Autodesk Inventor part; units mm, degrees
ref_plane "YZ Plane" through (0, 0, 0) normal (1, 0, 0) x (0, 1, 0)
ref_plane "XZ Plane" through (0, 0, 0) normal (0, 1, 0) x (-1, 0, 0)
ref_plane "XY Plane" through (0, 0, 0) normal (0, 0, 1) x (1, 0, 0)
sketch "Sketch1" plane through (0, 0, 0) normal (0, 0, 1) x (1, 0, 0)
  line L0 (-21.6696, 43.0812) -> (79.9304, 43.0812)
  line L1 (79.9304, 43.0812) -> (79.9304, -20.4188)
  line L2 (79.9304, -20.4188) -> (-21.6696, -20.4188)
  line L3 (-21.6696, -20.4188) -> (-21.6696, 43.0812)
  point P0 (0, 0)
  dimension "d0" = 101.6
  dimension "d1" = 63.5
extrude "Extrusion1" add sketch "Sketch1" along normal blind 7.9375
sketch "Sketch3" plane through (0, 0, 7.9375) normal (0, 0, 1) x (1, 0, 0)
  line L0 (-21.6696, 43.0812) -> (79.9304, 43.0812)
  line L1 (-21.6696, -20.4188) -> (-21.6696, 43.0812)
  point P0 (0, 0)
  point P1 (29.1304, 11.3312)
  dimension "d15" = 31.75
  dimension "d16" = 50.8
hole "Hole2" at (29.1304, 11.3312, 7.9375) direction (0, 0, -1) diameter 50.8 end through all
sketch "Sketch4" plane through (0, 0, 7.9375) normal (0, 0, 1) x (1, 0, 0)
  line L0 (-21.6696, -20.4188) -> (-21.6696, 43.0812)
  line L1 (79.9304, -20.4188) -> (-21.6696, -20.4188)
  point P0 (0, 0)
  point P1 (10.0804, 36.7312)
  point P2 (10.0804, -14.0688)
  point P3 (48.1804, 36.7312)
  point P4 (48.1804, -14.0688)
  dimension "d24" = 50.8
  dimension "d25" = 6.35
  dimension "d26" = 38.1
  dimension "d27" = 31.75
  dimension "d28" = 31.75
hole "Hole3" at (10.0804, 36.7312, 7.9375) at (10.0804, -14.0688, 7.9375) at (48.1804, 36.7312, 7.9375) at (48.1804, -14.0688, 7.9375) direction (0, 0, -1) diameter 3.9624 end through all
sketch "Sketch5" plane through (0, 0, 7.9375) normal (0, 0, 1) x (1, 0, 0)
  line L0 (79.9304, 43.0812) -> (79.9304, -20.4188)
  line L1 (-21.6696, 43.0812) -> (79.9304, 43.0812)
  line L2 (-21.6696, -20.4188) -> (-21.6696, 43.0812)
  line L3 (79.9304, -20.4188) -> (-21.6696, -20.4188)
  point P0 (0, 0)
  point P1 (-18.1136, 39.5252)
  point P2 (-18.1136, -16.8628)
  point P3 (76.3744, -16.8628)
  point P4 (76.3744, 39.5252)
  point P5 (-18.1136, 11.3312)
  point P6 (76.3744, 11.3312)
  dimension "d36" = 3.556
  dimension "d37" = 3.556
  dimension "d38" = 3.556
  dimension "d39" = 3.556
  dimension "d47" = 3.556
  dimension "d48" = 3.556
  dimension "d49" = 3.556
  dimension "d50" = 3.556
  dimension "d51" = 3.556
  dimension "d52" = 3.556
  dimension "d66" = 94.488
  dimension "d67" = 56.388
hole "Hole4" at (-18.1136, 39.5252, 7.9375) at (-18.1136, -16.8628, 7.9375) at (76.3744, -16.8628, 7.9375) at (76.3744, 39.5252, 7.9375) at (-18.1136, 11.3312, 7.9375) at (76.3744, 11.3312, 7.9375) direction (0, 0, -1) diameter 4.318 end through all counterbore diameter 6.985 counterbore depth 4.1656
sketch "Sketch6" plane through (0, 0, 7.9375) normal (0, 0, 1) x (1, 0, 0)
  line L0 (79.9304, 43.0812) -> (79.9304, -20.4188)
  line L1 (-21.6696, 43.0812) -> (79.9304, 43.0812)
  line L2 (-21.6696, -20.4188) -> (-21.6696, 43.0812)
  line L3 (79.9304, -20.4188) -> (-21.6696, -20.4188)
  point P0 (0, 0)
  point P1 (-8.9696, 30.3812)
  point P2 (-8.9696, -7.7188)
  point P3 (67.2304, 30.3812)
  point P4 (67.2304, -7.7188)
  dimension "d53" = 12.7
  dimension "d54" = 12.7
  dimension "d55" = 12.7
  dimension "d56" = 12.7
  dimension "d64" = 12.7
  dimension "d65" = 12.7
hole "Hole5" at (-8.9696, 30.3812, 7.9375) at (-8.9696, -7.7188, 7.9375) at (67.2304, 30.3812, 7.9375) at (67.2304, -7.7188, 7.9375) direction (0, 0, -1) diameter 6.4008 end through all
properties part number "JF-AT-JC0014" material "Aluminum-6061 (Anodized Black)"
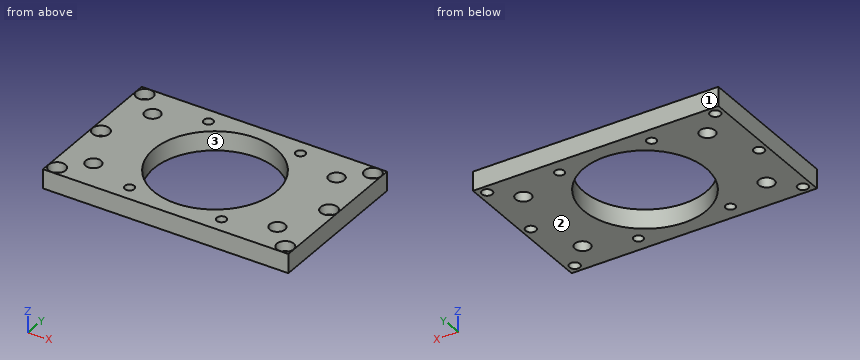
Model file for the job. Use its own axes, mm. Face numbers are marked on the shaded views. Give positions to 0.01 mm unless a question says otherwise; leave off trailing zeros. Order: outer loops, then holes, each group sorted by start corner. A loop starts at its lowest first (then second) coordinate and runs counter-clockwise, first axis right, second up. Notation, with made-up numbers: M 16,-7.75 L 23,-7.75 A12 cw 23,3.25 Z; hole C 9,88 d3. An arc over 180 degrees is marked long. Put each result on its own line as item: value. Start each with the question number.
(1) Pull direction Y, two halves, no side cores. Call the marked faces 1, 2 and 3: released by +Y, released by -Y, zero draft, split by the parting line, or undercut.
(2) Band-saw the part on A-A on y = 11.5. Give the cut face in (x, z).
(3) Band-saw the part on C-C on x = 24. Give the cut face in (y, z).
(4) Band-saw the part on B-B on z = 5.25. Count the separate pieces of the cut face and the enclosed holes in it, then the cut area to 3 significant figures.
(5) Band-saw the part on D-D on y = 20.5. Give the cut face in (x, z).
(6) Pin check, flat tips, straight feed: pin 1 Ø2 at (x, y) = (77.5, -15) entering from +Z; pin 2 Ø3 at (x, y) = (10.08, 36.73) entering from -Z. Stop position of each tip, or through.
(7) Drill centre lines: L1, parallel to X at y = 9, z = 7; L2, parallel to X at y = -15, z = 5.5; L3, parallel to X at y = -5.5, z = 1. Where is each one in solid material? Low to high. Write a range as [from, to].
Results below:
1. face 1: released by +Y
1. face 2: zero draft
1. face 3: undercut
2. outline: M -21.67,0 L -20.27,0 L -20.27,3.77 L -21.6,3.77 L -21.6,7.94 L -21.67,7.94 Z; M -15.96,0 L 3.73,0 L 3.73,7.94 L -14.63,7.94 L -14.63,3.77 L -15.96,3.77 Z; M 54.53,0 L 74.22,0 L 74.22,3.77 L 72.89,3.77 L 72.89,7.94 L 54.53,7.94 Z; M 78.53,0 L 79.93,0 L 79.93,7.94 L 79.86,7.94 L 79.86,3.77 L 78.53,3.77 Z
3. outline: M -20.42,0 L -13.55,0 L -13.55,7.94 L -20.42,7.94 Z; M 36.21,0 L 43.08,0 L 43.08,7.94 L 36.21,7.94 Z
4. separate pieces: 1
4. enclosed holes: 15
4. area: 4,020 mm2
5. outline: M -21.67,0 L 5.44,0 L 5.44,7.94 L -21.67,7.94 Z; M 52.82,0 L 79.93,0 L 79.93,7.94 L 52.82,7.94 Z
6. pin 1: stops at z = 3.77
6. pin 2: passes through
7. L1: x = [-21.67, -20.71], [-15.51, 3.84], [54.42, 73.77], [78.97, 79.93]
7. L2: x = [-21.67, -21.07], [-15.16, 8.33], [11.83, 46.43], [49.93, 73.42], [79.33, 79.93]
7. L3: x = [-21.67, -11.28], [-6.66, 10.11], [48.15, 64.92], [69.54, 79.93]
